from build123d import *

# Parameters (mm, degrees)
SKETCH2_R           = 50
SKETCH2_R_2         = 45
BOSS_EXTRUDE3_DEPTH = 200
SKETCH4_W           = 105
SKETCH4_H           = 105
BOSS_EXTRUDE5_DEPTH = 10


with BuildPart() as part:
    # Sketch2 → Boss-Extrude3 (new body)
    with BuildSketch(Plane(origin=(0, 0, 0), x_dir=(1, 0, 0), z_dir=(0, 1, 0))):
        Circle(SKETCH2_R)
        Circle(SKETCH2_R_2, mode=Mode.SUBTRACT)
    extrude(amount=BOSS_EXTRUDE3_DEPTH)

    # Sketch4 → Boss-Extrude5 (add)
    with BuildSketch(Plane(origin=(0, 0, 0), x_dir=(1, 0, 0), z_dir=(0, 1, 0))):
        Rectangle(SKETCH4_W, SKETCH4_H)
    extrude(amount=-BOSS_EXTRUDE5_DEPTH)


solid = part.part
Read the model definition and answer for the solid it produces. Units are mm, in the model's axes. A direction names the side the tool comes from. Coordinates: 2 decimals unless noted, no trailing zeros. Loops run counter-clockwise (first coordinate to the right, second up) from the corner with the lowest first, then second, coordinate; pieces in that order, holes last.
Q1. The part is cut by section A-A on x = 0. Write down the section's boundary in (y, z).
Q2. Which of the six approach directions +Z, -Z, +X, -X, +Y, -Y give full straight-line access (tool end or side, diameter ignored) to faces 4 (the face through (-1, -5, -52.5)), 5 (the face through (-1, 0, -1))?
Q3. The part is cut by section B-B on z = 0. Write down the section's boundary in (x, y).
Q4. The part is cut by section C-C on y = 4. Write down the section's boundary in (x, z), and give its area (3 significant figures).
Q5. The mould has two halves that part along Z. Classify faces 1 (the face through (-1, -10, -1)), 2 (the face through (-1, -5, 52.5)), 3 (the face through (20.765, 98.6, 39.923)): +Z half, -Z half, draft (parallel to the pull), parting line (faces both ways), or undercut.
Q6. Each of these flat-tipped pins is pushed along its axis until it touches: pin 1 Ø10 at (x, y) = (-41.5, 107.5) entering from -Z; pin 2 Ø6 at (x, y) = (11.5, 55.5) entering from -Z; pin 3 Ø12 at (y, z) = (23, -4) entering from +X. Where does it stop, or does it pass through?
Q7. Consider probe 1 along X at (y, z) = (115, 0); probe 2 along Y at (x, z) = (-15, -31). Determine where each line is inside the solid, lowest interval first.
Results below:
1. outline: (-10, -52.5) - (0, -52.5) - (0, -50) - (200, -50) - (200, -45) - (0, -45) - (0, 45) - (200, 45) - (200, 50) - (0, 50) - (0, 52.5) - (-10, 52.5) - close
2. face 4: -Z, +X, -X, +Y, -Y
2. face 5: +Y
3. outline: (-52.5, -10) - (52.5, -10) - (52.5, 0) - (50, 0) - (50, 200) - (45, 200) - (45, 0) - (-45, 0) - (-45, 200) - (-50, 200) - (-50, 0) - (-52.5, 0) - close
4. outline: circle Ø100 at (0, 0); hole circle Ø90 at (0, 0)
4. area: 1,490 mm2
5. face 1: draft
5. face 2: +Z half
5. face 3: undercut
6. pin 1: stops at z = -34.17
6. pin 2: stops at z = -49.27
6. pin 3: stops at x = 50
7. probe 1: x = -50 to -45, 45 to 50
7. probe 2: y = -10 to 0
